Geometry: see drawing. Coordinates: mm, zero at the bounding-box minimum. A direction names the side the tool comes from. Give positions to 0.01 mm unless a question says otherwise; leave off trailing zeros. Write each loop counter-clockwise with the first axis right and the second up, starting at its lowest first coordinate (ties: lowest second). Pieces come first, ordered by that corner, then holes. Notation, with made-up numbers: (-11, 2) - (47, 2) arc R8 ccw to (47, 16) - close; hole circle Ø9 at (57.25, 87.5). An arc over 180 degrees is marked (long way). Return JSON: item names as keys, results as strings.
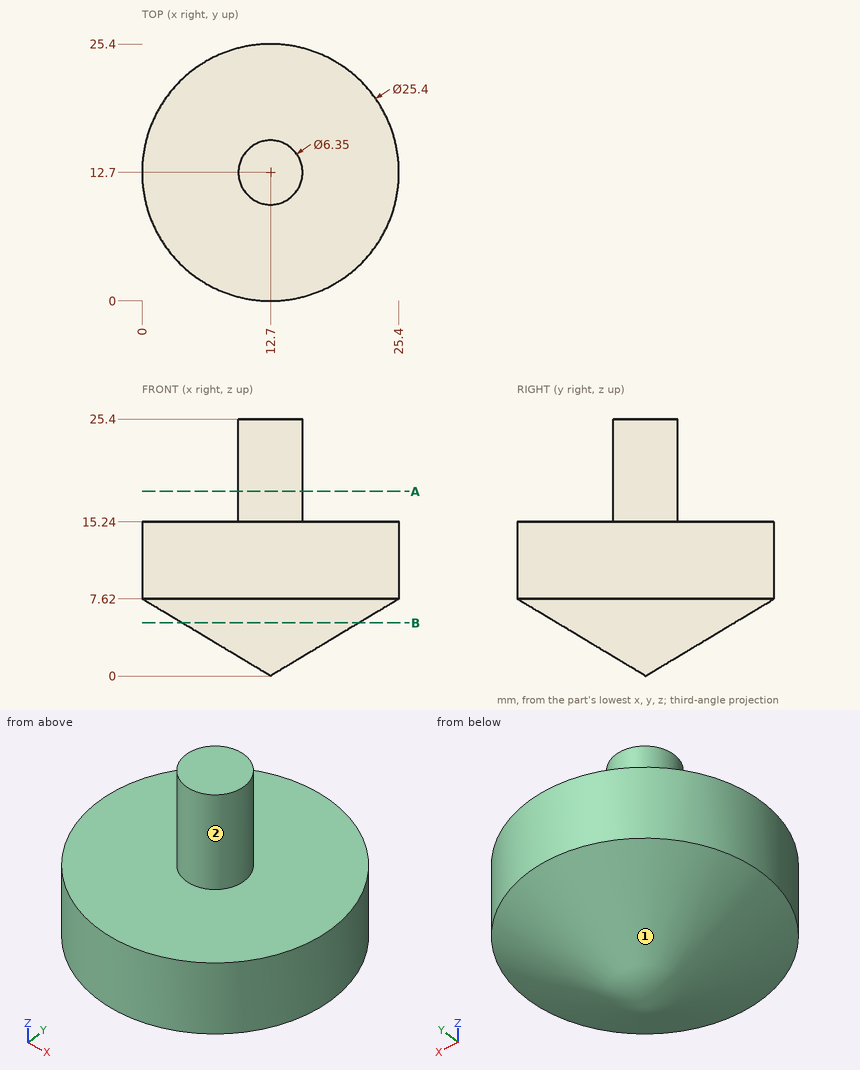
Q1. Set-up query: the marked faces 1 and 2. Return all of +Z, -Z, +X, -X, +Y, -Y with unobstructed straight access to the full face (end or side cutting, diameter ignored); none if empty.
Answer key:
{"face 1": "-Z", "face 2": "+Z"}
Q2. Material intervals for probe 1 along X at (y, z) = (12.5, 19.75); probe 2 along Y at (x, z) = (10, 13.75); probe 3 along Y at (x, z) = (6.5, 7.5), sorted ascending. Write a range as [from, to].
Answer key:
{"probe 1": "x = [9.53, 15.87]", "probe 2": "y = [0.29, 25.11]", "probe 3": "y = [1.85, 23.55]"}
Q3. Section query B-B, the plane z = 5.25. Return the cut outline in (x, y), plus the area to 3 significant figures.
Answer key:
{"outline": "circle Ø17.5 at (12.7, 12.7)", "area": "241 mm^2"}
Q4. Section query A-A, the plane z = 18.25. Return the cut outline in (x, y) (3 decimals), plus the area to 3 significant figures.
Answer key:
{"outline": "circle Ø6.35 at (12.7, 12.7)", "area": "31.7 mm^2"}
Q5. Pin query (flat end, axial travel): P1, Ø3, axis at x = 15, y = 18.5, coming from the -Z side; P2, Ø1, axis at x = 10.5, z = 20.5, coming from the +Y side; P3, Ø1, axis at x = 5, y = 14, coming from the +Z side. Return the tip coordinate at first contact, or that it passes through.
Answer key:
{"P1": "stops at z = 2.84", "P2": "stops at y = 15.38", "P3": "stops at z = 15.24"}
